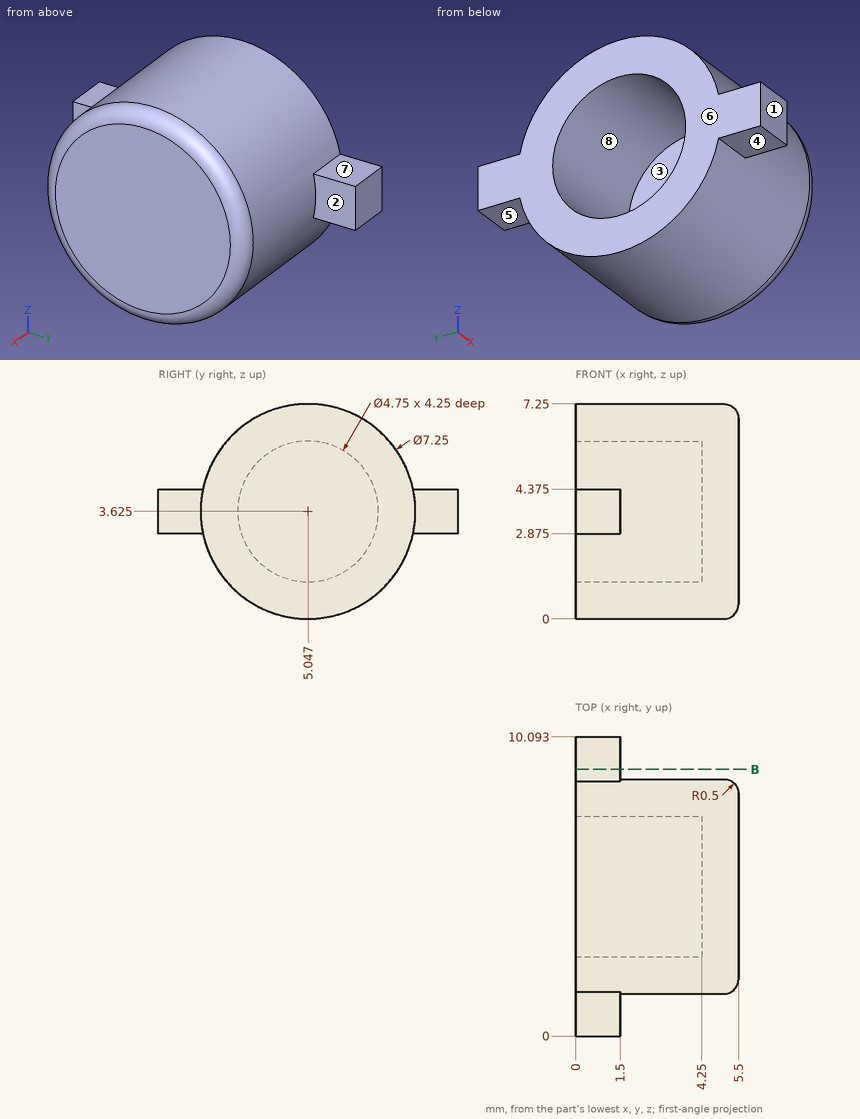
Check sheet for the drawn part. Datum: minimum x, y, z corner. Units: mm. A direction names the side the tool comes from. Coordinates: 2 decimals unless noted, no trailing zeros. Write each loop counter-clockwise with the first axis right and the second up, starting at its lowest first coordinate (ties: lowest second). Pieces come first, ordered by that corner, then holes. Notation, with made-up numbers: (-8.75, 32.5) - (27.25, 32.5) arc R25 cw to (27.25, 61.5) - close; hole circle Ø5 at (42.25, 89). An arc over 180 degrees is marked (long way). Answer as a JSON object with one key per item and string values.
(1) Gauge pin test, flat ends, axial feed: pin 1 Ø1.2 at (x, y) = (1, 0.5) entering from +Z (3 decimals); pin 2 Ø2 at (x, y) = (2.5, 7.5) entering from -Z (1 decimal); pin 3 Ø2 at (y, z) = (5.5, 3) entering from -X. Record the tip position at first contact, or that the pin passes through.
Report:
{"pin 1": "z = 4.375", "pin 2": "z = 0.3", "pin 3": "x = 4.25"}
(2) Mould release check, pull along Y, two halves, no side actions. Record for the marked faces 1, 2 and 3: pulls with the +Y half, pulls with the -Y half, needs draft (parallel to the pull), parting line crosses it, or undercut.
Report:
{"face 1": "pulls with the -Y half", "face 2": "needs draft", "face 3": "undercut"}
(3) Thickness scan on line 1 along Z through (x, y) = (0.9, 8.75) (1 decimal); line 2 along Y through (x, z) = (1.85, 3.75) (1 decimal); line 3 along X through (y, z) = (6.5, 4.75). Record the ranges inside material, lowest first.
Report:
{"line 1": "2.9 to 4.4", "line 2": "1.4 to 2.7, 7.4 to 8.7", "line 3": "4.25 to 5.5"}
(4) Cross-section at B-B on y = 9. Record the cut outline in (x, z) (1 decimal).
Report:
{"outline": "(0, 2.9) - (1.5, 2.9) - (1.5, 4.4) - (0, 4.4) - close"}
(5) Tool access check on the marked faces 4, 5, 6, 7 and 8. Record the directions out of +Z, -Z, +X, -X, +Y, -Y that give a thin tool (end or side, any length) a straight path to the whole face; none if there is none.
Report:
{"face 4": "-Z, +X, -X, -Y", "face 5": "-Z, +X, -X, +Y", "face 6": "+Z, -Z, -X, +Y, -Y", "face 7": "+Z, +X, -X, +Y", "face 8": "-X"}
